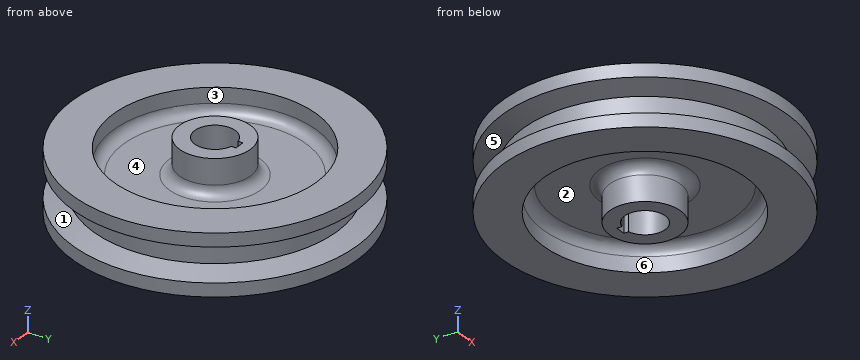
from build123d import *

# Parameters (mm, degrees)
SKETCH2_W          = 0.25
SKETCH2_H          = 0.370788844
CUT_EXTRUDE1_DEPTH = 20.6248


with BuildPart() as part:
    # Sketch1 → Revolve1 (revolve)
    with BuildSketch(Plane(origin=(0, 0, 0), x_dir=(0, 0, -1), z_dir=(1, 0, 0))):
        with BuildLine():
            Line((1, 0.875), (0.375, 0.875))
            ThreePointArc((0.375, 0.875), (0.198223305, 0.948223305), (0.125, 1.125))
            Line((0.125, 1.125), (0.125, 2.25))
            ThreePointArc((0.125, 2.25), (0.198223305, 2.426776695), (0.375, 2.5))
            Line((0.375, 2.5), (0.75, 2.5))
            Line((0.75, 2.5), (0.75, 3.5))
            Line((0.75, 3.5), (0.42, 3.5))
            Line((0.42, 3.5), (0.25, 3))
            Line((0.25, 3), (-0.25, 3))
            Line((-0.25, 3), (-0.42, 3.5))
            Line((-0.42, 3.5), (-0.75, 3.5))
            Line((-0.75, 3.5), (-0.75, 2.5))
            Line((-0.75, 2.5), (-0.375, 2.5))
            ThreePointArc((-0.375, 2.5), (-0.198223305, 2.426776695), (-0.125, 2.25))
            Line((-0.125, 2.25), (-0.125, 1.125))
            ThreePointArc((-0.125, 1.125), (-0.198223305, 0.948223305), (-0.375, 0.875))
            Line((-0.375, 0.875), (-1, 0.875))
            Line((-1, 0.875), (-1, 0.5))
            Line((-1, 0.5), (1, 0.5))
            Line((1, 0.5), (1, 0.875))
        make_face()
    revolve(axis=Axis((0, 0, 1.479906814), (0, 0, -1)))

    # Sketch2 → Cut-Extrude1 (cut)
    with BuildSketch(Plane.XY.offset(1)):
        with Locations((0, 0.414605578)):
            Rectangle(SKETCH2_W, SKETCH2_H)
    extrude(amount=-CUT_EXTRUDE1_DEPTH, mode=Mode.SUBTRACT)


solid = part.part
Geometry: final body of the model. Coordinates: model frame, mm. Face numbers are marked on the shaded views. A direction names the side the tool comes from. Round coordinates to 2 decimals unless told otherwise and drop trailing zeros. Loops run counter-clockwise (first coordinate to the right, second up) from the corner with the lowest first, then second, coordinate; pieces in that order, holes last. Notation, with made-up numbers: M 75,-2.5 L 115,-2.5 A20 cw 115,34.5 Z; hole C 25,-38.75 d4. An arc over 180 degrees is marked long. One line per question, with ' | ' between items.
(1) Access query for the marked faces 1, 2 and 3. Directions: +Z, -Z, +X, -X, +Y, -Y. A direction counts if a zero-diameter tool reaches every point of the face in a straight line with its end or side. Return the directions, or none.
Check result:
face 1: none | face 2: -Z | face 3: +Z
(2) Contact query for flat-ended pins moving along their axis: P1, Ø1, axis at x = -1.5, z = -0.5, coming from the -Y side; P2, Ø2, axis at x = -1.5, y = -2, coming from the +Z side; P3, Ø1, axis at y = 1.5, z = 0, coming from the -X side. Output: stop coordinate, or through.
Check result:
P1: stops at y = -3.35 | P2: stops at z = 0.75 | P3: stops at x = -3.28
(3) Pull-direction query (Z, two-part tool) for the marked faces 4, 5 and 6; classes: +Z half, -Z half, draft (parallel to the pull), parting line (faces both ways), or undercut.
Check result:
face 4: +Z half | face 5: undercut | face 6: draft
(4) Material intervals for line 1 along X through (y, z) = (0, -0.5) (3 decimals); line 2 along X through (y, z) = (0, -0.2); line 3 along Z through (x, y) = (0, 1.25) (3 decimals), sorted ascending. Write a range as from..to.
Check result:
line 1: x = -3.5..-2.5, -0.875..-0.5, 0.5..0.875, 2.5..3.5 | line 2: x = -3..-2.43, -0.95..-0.5, 0.5..0.95, 2.43..3 | line 3: z = -0.125..0.125
(5) Cut plane A-A on z = -0.55. Return the cut outline in (x, y) (3 decimals).
Check result:
outline: C 0,0 d7; C 0,0 d1.75; hole C 0,0 d5; hole M -0.125,0.484 A0.5 ccw long 0.125,0.484 L 0.125,0.6 L -0.125,0.6 Z
